from build123d import *

# Parameters (mm, degrees)
SKETCH1_W           = 91
SKETCH1_H           = 91
BOSS_EXTRUDE1_DEPTH = 0.5
SKETCH2_W           = 77
SKETCH2_H           = 77
BOSS_EXTRUDE2_DEPTH = 10
FILLET1_R           = 5
CUT_EXTRUDE1_DEPTH  = 66.119121616
FILLET2_R           = 10
BOSS_EXTRUDE3_START = 0.5
SKETCH7_R           = 35
BOSS_EXTRUDE3_DEPTH = 0.5


with BuildPart() as part:
    # Sketch1 → Boss-Extrude1 (new body)
    with BuildSketch(Plane.XY):
        Rectangle(SKETCH1_W, SKETCH1_H)
    extrude(amount=BOSS_EXTRUDE1_DEPTH)

    # Sketch2 → Boss-Extrude2 (add)
    with BuildSketch(Plane.XY):
        Rectangle(SKETCH2_W, SKETCH2_H)
    extrude(amount=BOSS_EXTRUDE2_DEPTH)

    # Fillet1
    fillet1_edges = [part.edges().sort_by_distance(p)[0] for p in [
        (38.5, -38.5, 5.25),
        (38.5, 38.5, 5.25),
        (-38.5, 38.5, 5.25),
        (-38.5, -38.5, 5.25),
    ]]
    fillet(fillet1_edges, radius=FILLET1_R)

    # Sketch4 → Cut-Extrude1 (cut, through all)
    with BuildSketch(Plane.XY.offset(10)):
        with BuildLine():
            Line((-33.5, -37.5), (33.5, -37.5))
            ThreePointArc((33.5, -37.5), (36.328427125, -36.328427125), (37.5, -33.5))
            Line((37.5, -33.5), (37.5, 33.5))
            ThreePointArc((37.5, 33.5), (36.328427125, 36.328427125), (33.5, 37.5))
            Line((33.5, 37.5), (-33.5, 37.5))
            ThreePointArc((-33.5, 37.5), (-36.328427125, 36.328427125), (-37.5, 33.5))
            Line((-37.5, 33.5), (-37.5, -33.5))
            ThreePointArc((-37.5, -33.5), (-36.328427125, -36.328427125), (-33.5, -37.5))
        make_face()
    extrude(amount=-CUT_EXTRUDE1_DEPTH, mode=Mode.SUBTRACT)

    # Fillet2
    fillet2_edges = [part.edges().sort_by_distance(p)[0] for p in [
        (45.5, -45.5, 0.25),
        (-45.5, -45.5, 0.25),
        (-45.5, 45.5, 0.25),
        (45.5, 45.5, 0.25),
    ]]
    fillet(fillet2_edges, radius=FILLET2_R)

    # Sketch7 → Boss-Extrude3 (add)
    with BuildSketch(Plane.XY.offset(BOSS_EXTRUDE3_START)):
        with BuildLine():
            Line((-33.5, -37.5), (33.5, -37.5))
            ThreePointArc((33.5, -37.5), (36.328427125, -36.328427125), (37.5, -33.5))
            Line((37.5, -33.5), (37.5, 33.5))
            ThreePointArc((37.5, 33.5), (36.328427125, 36.328427125), (33.5, 37.5))
            Line((33.5, 37.5), (-33.5, 37.5))
            ThreePointArc((-33.5, 37.5), (-36.328427125, 36.328427125), (-37.5, 33.5))
            Line((-37.5, 33.5), (-37.5, -33.5))
            ThreePointArc((-37.5, -33.5), (-36.328427125, -36.328427125), (-33.5, -37.5))
        make_face()
        with Locations(Location((0, 0, 0), (0, 0, 180))):
            Circle(SKETCH7_R, mode=Mode.SUBTRACT)
    extrude(amount=-BOSS_EXTRUDE3_DEPTH)


solid = part.part
Verification items for the finished model (mm, model axes). A direction names the side the tool comes from. Round coordinates to 2 decimals unless told otherwise and drop trailing zeros. Write each loop counter-clockwise with the first axis right and the second up, starting at its lowest first coordinate (ties: lowest second). Pieces come first, ordered by that corner, then holes.
(1) Mould release check, pull along Y, two halves, no side actions. Record for faces 1 (the cylindrical face through (-42.65, -42.49, 0.25)), 2 (the flat face through (0, -37.5, 5)), 3 (the flat face through (20, 31, 0)), 4 (the cylindrical face through (-42.65, 42.49, 0.25)): pulls with the +Y half, pulls with the -Y half, needs draft (parallel to the pull), parting line crosses it, or undercut.
Returned:
face 1: pulls with the -Y half
face 2: undercut
face 3: needs draft
face 4: pulls with the +Y half
(2) Access from +Z, -Z, +X, -X, +Y, -Y to the whole of each face (thin tool, end or side, straight path). Record for faces 5 (the flat face through (0, 38.5, 5)), 6 (the cylindrical face through (-36.297, 36.359, 5.316)), 7 (the cylindrical face through (37, -37.07, 5.32)), 8 (the flat face through (-38.5, 0, 5)).
Returned:
face 5: +Z, +X, -X, +Y
face 6: +Z
face 7: +Z, +X, -Y
face 8: +Z, -X, +Y, -Y
(3) Section check B-B (z = 7.25). Enter the section's corners in (x, y), plus the area to 3 significant figures.
Returned:
outline: (-38.5, -33.5) arc R5 ccw to (-33.5, -38.5) - (33.5, -38.5) arc R5 ccw to (38.5, -33.5) - (38.5, 33.5) arc R5 ccw to (33.5, 38.5) - (-33.5, 38.5) arc R5 ccw to (-38.5, 33.5) - close; hole (-37.5, -33.5) arc R4 ccw to (-33.5, -37.5) - (33.5, -37.5) arc R4 ccw to (37.5, -33.5) - (37.5, 33.5) arc R4 ccw to (33.5, 37.5) - (-33.5, 37.5) arc R4 ccw to (-37.5, 33.5) - close
area: 296 mm2
(4) Section check A-A (y = 0). Enter the section's corners in (x, z).
Returned:
outline: (-45.5, 0) - (-35, 0) - (-35, 0.5) - (-37.5, 0.5) - (-37.5, 10) - (-38.5, 10) - (-38.5, 0.5) - (-45.5, 0.5) - close; (35, 0) - (45.5, 0) - (45.5, 0.5) - (38.5, 0.5) - (38.5, 10) - (37.5, 10) - (37.5, 0.5) - (35, 0.5) - close
(5) Section check D-D (x = 40.5). Enter the section's corners in (y, z), plus the area to 3 significant figures.
Returned:
outline: (-44.16, 0) - (44.16, 0) - (44.16, 0.5) - (-44.16, 0.5) - close
area: 44.2 mm2
(6) Material ranges on line 1 (X direction, y = 13, z = 2.75); line 2 (Y direction, x = 0, z = 0.1), recorded low to high.
Returned:
line 1: x = -38.5 to -37.5, 37.5 to 38.5
line 2: y = -45.5 to -35, 35 to 45.5
(7) Section check C-C (x = -28). Enter the section's corners in (y, z).
Returned:
outline: (-45.5, 0) - (-21, 0) - (-21, 0.5) - (-37.5, 0.5) - (-37.5, 10) - (-38.5, 10) - (-38.5, 0.5) - (-45.5, 0.5) - close; (21, 0) - (45.5, 0) - (45.5, 0.5) - (38.5, 0.5) - (38.5, 10) - (37.5, 10) - (37.5, 0.5) - (21, 0.5) - close
(8) Depth check by flat-ended pin: pin 1 Ø3 at (y, z) = (17.5, 3.5) entering from +X; pin 2 Ø1 at (y, z) = (26.5, 2.5) entering from -X; pin 3 Ø2 at (x, z) = (-1.5, 4.5) entering from -Y; pin 4 Ø8 at (x, y) = (5, 27) entering from +Z. Enter the tip coordinate at first touch or a pass-through.
Returned:
pin 1: stops at x = 38.5
pin 2: stops at x = -38.5
pin 3: stops at y = -38.5
pin 4: passes through
